from build123d import *

# Parameters (mm, degrees)
SKETCH6_W               = 15
SKETCH6_H               = 38
CUT_EXTRUDE3_DEPTH      = 21
CUT_EXTRUDE3_DEPTH_BACK = 21
SKETCH10_W              = 17.380716029
SKETCH10_H              = 23.242829716
CUT_EXTRUDE4_DEPTH      = 21
CUT_EXTRUDE4_DEPTH_BACK = 21
SKETCH11_R              = 4.5
CUT_EXTRUDE5_DEPTH      = 13.540496218
CUT_EXTRUDE5_DEPTH_BACK = 25.540496218
SKETCH12_R              = 4.5
CUT_EXTRUDE6_DEPTH      = 21
CUT_EXTRUDE6_DEPTH_BACK = 21


with BuildPart() as part:
    # Sketch1 → Revolve1 (revolve)
    with BuildSketch(Plane.XY):
        with BuildLine():
            Line((-13.869223911, 45.909090909), (-19.813177016, 2.727272727))
            ThreePointArc((-19.813177016, 2.727272727), (-15.075567229, -13.142574813), (0, -20))
            Line((0, -20), (0, 58))
            ThreePointArc((0, 58), (-9.199802369, 54.55289706), (-13.869223911, 45.909090909))
        make_face()
    revolve(axis=Axis((0, 58, 0), (0, -1, 0)))

    # Sketch6 → Cut-Extrude3 (cut, two sides)
    with BuildSketch(Plane.XY) as cut_extrude3_sk:
        with Locations((0, -1)):
            Rectangle(SKETCH6_W, SKETCH6_H)
    extrude(amount=CUT_EXTRUDE3_DEPTH, mode=Mode.SUBTRACT)
    extrude(cut_extrude3_sk.sketch, amount=-CUT_EXTRUDE3_DEPTH_BACK, mode=Mode.SUBTRACT)

    # Sketch10 → Cut-Extrude4 (cut, two sides)
    with BuildSketch(Plane(origin=(0, 0, 0), x_dir=(0, 0, -1), z_dir=(1, 0, 0))) as cut_extrude4_sk:
        with Locations((-14.690358015, 45.212221832)):
            Rectangle(SKETCH10_W, SKETCH10_H)
        with Locations((14.690358015, 45.212221832)):
            Rectangle(SKETCH10_W, SKETCH10_H)
    extrude(amount=CUT_EXTRUDE4_DEPTH, mode=Mode.SUBTRACT)
    extrude(cut_extrude4_sk.sketch, amount=-CUT_EXTRUDE4_DEPTH_BACK, mode=Mode.SUBTRACT)

    # Sketch11 → Cut-Extrude5 (cut, two sides)
    with BuildSketch(Plane(origin=(0, 0, -6), x_dir=(-1, 0, 0), z_dir=(0, 0, -1))) as cut_extrude5_sk:
        with Locations((0, 44)):
            Circle(SKETCH11_R)
    extrude(amount=CUT_EXTRUDE5_DEPTH, mode=Mode.SUBTRACT)
    extrude(cut_extrude5_sk.sketch, amount=-CUT_EXTRUDE5_DEPTH_BACK, mode=Mode.SUBTRACT)

    # Sketch12 → Cut-Extrude6 (cut, two sides)
    with BuildSketch(Plane(origin=(0, 0, 0), x_dir=(0, 0, -1), z_dir=(1, 0, 0))) as cut_extrude6_sk:
        Circle(SKETCH12_R)
    extrude(amount=CUT_EXTRUDE6_DEPTH, mode=Mode.SUBTRACT)
    extrude(cut_extrude6_sk.sketch, amount=-CUT_EXTRUDE6_DEPTH_BACK, mode=Mode.SUBTRACT)


solid = part.part
Model file for the job. Use its own axes, mm. A direction names the side the tool comes from. Coordinates: 2 decimals unless noted, no trailing zeros. Loops run counter-clockwise (first coordinate to the right, second up) from the corner with the lowest first, then second, coordinate; pieces in that order, holes last. Notation, with made-up numbers: (-2, 8.25) -> (19, 8.25) arc R13 ccw to (19, 33.25) -> close; hole circle Ø3 at (64, 2.25). An arc over 180 degrees is marked (long way). Use one line per item in the form item = value. Start each with the question number.
(1) Cut at D-D on y = 13. Give the cut face in (x, z).
(2) Tool access for faces 5 (the cylindrical face through (-13.45, 4.46, 0.59)), 6 (the flat face through (3, 40, -6)), 7 (the flat face through (0, 33.591, 10)), 8 (the flat face through (7.5, 4, -4)): list every direction of +Z, -Z, +X, -X, +Y, -Y with a clear straight run to the whole face (end or side of a thin tool).
(3) Flat gauge pins, fed straight in: pin 1 (16.5 mm diameter, centred on x = -1, z = 0, fed in from -Y); pin 2 (14.5 mm diameter, centred on x = 0, y = 44, fed in from +Z); pin 3 (1.5 mm diameter, centred on x = 10, y = 17.5, fed in from -Z). Where does each tip first touch, or does it go through?
(4) Cut at C-C on y = 44. Give the cut face in (x, z), and give its area (3 significant figures).
(5) Probe probe 1 along X at (y, z) = (7.5, 12.5); probe 2 along Y at (x, z) = (9, -3); probe 3 along Y at (x, z) = (3, -7). List the from-to ranges inside material, lowest first. Write a range as from..to.
(6) Cut at B-B on x = 0. Give the cut face in (y, z).
(7) Pull direction Y, two halves, no side cores. Call faces 1 (the flat face through (0, 33.591, -10)), 2 (the flat face through (-7.5, 4, -4)), 3 (the cylindrical face through (0.98, 39.61, -0.08)), 4 (the flat face through (0, 18, 0)): pulls with the +Y half, pulls with the -Y half, needs draft (parallel to the pull), parting line crosses it, or undercut.
(8) Cut at A-A on z = 0. Give the cut face in (x, y).
Values:
q1.outline = (-7.5, -16.8) -> (-7.5, 16.8) arc R18.4 ccw to start; (7.5, -16.8) arc R18.4 ccw to (7.5, 16.8) -> close
q2.face_5 = +X, -X
q2.face_6 = -Z, +X, -X, +Y
q2.face_7 = +Z, +X, -X, +Y
q2.face_8 = +Z, -Z, -Y
q3.pin_1 = -18.54
q3.pin_2 = 6
q3.pin_3 = -15.2
q4.outline = (-12.8, -6) -> (-4.5, -6) -> (-4.5, 6) -> (-12.8, 6) arc R14.13 ccw to start; (4.5, -6) -> (12.8, -6) arc R14.13 ccw to (12.8, 6) -> (4.5, 6) -> close
q4.area = 221 mm2
q5.probe_1 = -14.52..-7.5, 7.5..14.52
q5.probe_2 = -17.61..-3.35, 3.35..54.3
q5.probe_3 = 18..33.59
q6.outline = (18, -17.71) -> (33.59, -15.56) -> (33.59, -6) -> (39.5, -6) -> (39.5, 6) -> (33.59, 6) -> (33.59, 15.56) -> (18, 17.71) -> close; (48.5, -6) -> (56.65, -6) arc R14 ccw to (56.65, 6) -> (48.5, 6) -> close
q7.face_1 = pulls with the +Y half
q7.face_2 = needs draft
q7.face_3 = undercut
q7.face_4 = pulls with the -Y half
q8.outline = (-19.57, 4.5) -> (-7.5, 4.5) -> (-7.5, 18) -> (7.5, 18) -> (7.5, 4.5) -> (19.57, 4.5) -> (13.87, 45.91) arc R14 ccw to (-13.87, 45.91) -> close; (-19.49, -4.5) arc R20 ccw to (-7.5, -18.54) -> (-7.5, -4.5) -> close; (7.5, -18.54) arc R20 ccw to (19.49, -4.5) -> (7.5, -4.5) -> close; hole circle Ø9 at (0, 44)
